Here's how the part is built. I have some questions about the finished solid (model axes, mm). Face numbers are marked on the shaded views. Round coordinates to 2 decimals unless told otherwise and drop trailing zeros. Write each loop counter-clockwise with the first axis right and the second up, starting at its lowest first coordinate (ties: lowest second). Pieces come first, ordered by that corner, then holes. Notation, with made-up numbers: (58.5, 1) -> (96.5, 1) arc R27 ccw to (96.5, 34) -> close; hole circle Ø4 at (9.25, 87.5). An arc over 180 degrees is marked (long way). Put each result on its own line as item: value. Start each with the question number.
1. Suppose I cut it at D-D (x = 58). Please give me the cut outline in (y, z), then the cut area to 4 significant figures.
2. For pin 1 (12 mm diameter, centred on x = 8.5, z = 12.5, fed in from +Y); pin 2 (0.8 mm diameter, centred on y = -13.5, z = 2.5, fed in from +X); pin 3 (2 mm diameter, centred on y = -7, z = 1, fed in from -X); pin 4 (1 mm diameter, centred on y = -11, z = 8, fed in from +X), each with a flat end and sliding along its axis, tell me the tip position at first contact or that it passes through.
3. Suppose I cut it at B-B (x = 6). Please give me the cut outline in (y, z), then the cut area to 3 significant figures.
4. Suppose I cut it at A-A (y = -5). Please give me the cut outline in (x, z).
5. Suppose I cut it at C-C (z = 13.75). Please give me the cut outline in (x, y), then the cut area to 3 significant figures.
6. We'd pull the mould along Z, two halves only. Please class the marked faces 1, 2 and 3: +Z half, -Z half, draft (parallel to the pull), parting line (faces both ways), or undercut.
7. I need wall thicknesses on probe 1 along Z at (x, y) = (-17, -3.25); probe 2 along Y at (x, z) = (-31, 7.75); probe 3 along X at (y, z) = (-1, 19). Which ranges of each line are inside material? Lowest first, please. Write a range as from..to.
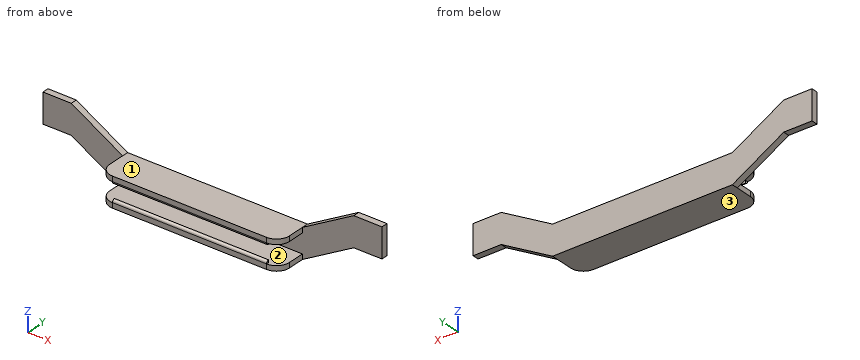
```python
from build123d import *

# Parameters (mm, degrees)
F0_W     = 70
F0_H     = 7.5
F1_DEPTH = 2.5
F0_H_2   = 2
F2_DEPTH = 14
F4_DEPTH = 30
F5_R     = 5


with BuildPart() as f1:
    # F0 (on Front) → F1 (new body)
    with BuildSketch(Plane.XZ):
        Polygon((-55, 23), (-66, 23), (-66, 11.5), (-55, 11.5), (-35, 0), (-35, 2), (-35, 9.5), (-35, 11.5), align=None)
        Polygon((55, 23), (35, 11.5), (35, 9.5), (35, 2), (35, 0), (55, 11.5), (66, 11.5), (66, 23), align=None)
        with Locations((0, 5.75)):
            Rectangle(F0_W, F0_H)
    extrude(amount=F1_DEPTH)

    # F0 (on Front) → F2 (join)
    with BuildSketch(Plane.XZ):
        with Locations((0, 10.5)):
            Rectangle(F0_W, F0_H_2)
        with Locations((0, 1)):
            Rectangle(F0_W, F0_H_2)
    extrude(amount=F2_DEPTH)

    # F3 (on Right) → F4 (join, symmetric)
    with BuildSketch(Plane.YZ):
        with BuildLine():
            Line((-13, 9.5), (-14, 9.5))
            ThreePointArc((-14, 9.5), (-13.7071067812, 8.7928932188), (-13, 8.5))
            Line((-13, 8.5), (-13, 9.5))
        make_face()
        with BuildLine():
            Line((-13, 2), (-13, 3))
            ThreePointArc((-13, 3), (-13.7071067812, 2.7071067812), (-14, 2))
            Line((-14, 2), (-13, 2))
        make_face()
    extrude(amount=F4_DEPTH, both=True)

    # F5
    f5_edges = [f1.edges().sort_by_distance(p)[0] for p in [
        (35, -14, 10.5),
        (35, -14, 1),
        (-35, -14, 1),
        (-35, -14, 10.5),
    ]]
    fillet(f5_edges, radius=F5_R)


solid = f1.part
```
Verdict:
1. outline: (-2.5, 11.5) -> (0, 11.5) -> (0, 23) -> (-2.5, 23) -> close
1. area: 28.75 mm^2
2. pin 1: stops at y = 0
2. pin 2: stops at x = 30
2. pin 3: stops at x = -35
2. pin 4: passes through
3. outline: (-14, 0) -> (0, 0) -> (0, 11.5) -> (-14, 11.5) -> (-14, 9.5) arc R1 ccw to (-13, 8.5) -> (-13, 9.5) -> (-2.5, 9.5) -> (-2.5, 2) -> (-13, 2) -> (-13, 3) arc R1 ccw to (-14, 2) -> close
3. area: 76.3 mm^2
4. outline: (-35, 0) -> (35, 0) -> (35, 2) -> (-35, 2) -> close; (-35, 9.5) -> (35, 9.5) -> (35, 11.5) -> (-35, 11.5) -> close
5. outline: (-66, -2.5) -> (-38.91, -2.5) -> (-38.91, 0) -> (-66, 0) -> close; (38.91, -2.5) -> (66, -2.5) -> (66, 0) -> (38.91, 0) -> close
5. area: 135 mm^2
6. face 1: +Z half
6. face 2: undercut
6. face 3: -Z half
7. probe 1: z = 0..2, 9.5..11.5
7. probe 2: y = -2.5..0
7. probe 3: x = -66..-48.04, 48.04..66
